from build123d import *

# Parameters (mm, degrees)
SKETCH_1_R      = 1.65
EXTRUDE_2_DEPTH = 2


with BuildPart() as part:
    # 草图1 → 凸台-拉伸2 (new body)
    with BuildSketch(Plane.XY):
        with BuildLine():
            ThreePointArc((64.930621202, 11.618442311), (61.467079618, -29.381557689), (64.930621202, -70.381557689))
            ThreePointArc((64.930621202, -70.381557689), (53.430621202, -81.881557689), (41.930621202, -70.381557689))
            ThreePointArc((41.930621202, -70.381557689), (45.394162787, -29.381557689), (41.930621202, 11.618442311))
            ThreePointArc((41.930621202, 11.618442311), (53.430621202, 23.118442311), (64.930621202, 11.618442311))
        make_face()
        with Locations((46.080621202, -70.381557689)):
            Circle(SKETCH_1_R, mode=Mode.SUBTRACT)
        with Locations((53.430621202, 4.268442311)):
            Circle(SKETCH_1_R, mode=Mode.SUBTRACT)
        with Locations((53.430621202, 11.618442311)):
            Circle(SKETCH_1_R, mode=Mode.SUBTRACT)
        with Locations((46.080621202, 11.618442311)):
            Circle(SKETCH_1_R, mode=Mode.SUBTRACT)
        with Locations((53.430621202, 18.968442311)):
            Circle(SKETCH_1_R, mode=Mode.SUBTRACT)
        with Locations((60.780621202, 11.618442311)):
            Circle(SKETCH_1_R, mode=Mode.SUBTRACT)
        with Locations((53.430621202, -70.381557689)):
            Circle(SKETCH_1_R, mode=Mode.SUBTRACT)
        with Locations((53.430621202, -63.031557689)):
            Circle(SKETCH_1_R, mode=Mode.SUBTRACT)
        with Locations((60.780621202, -70.381557689)):
            Circle(SKETCH_1_R, mode=Mode.SUBTRACT)
        with Locations((53.430621202, -77.731557689)):
            Circle(SKETCH_1_R, mode=Mode.SUBTRACT)
    extrude(amount=EXTRUDE_2_DEPTH)


solid = part.part
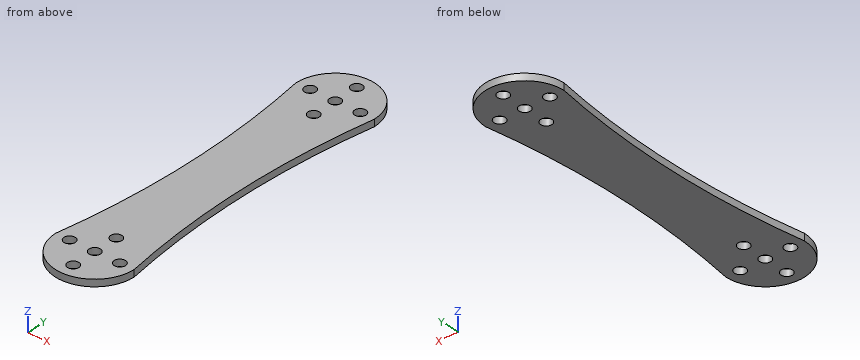
Geometry check sheet. Reference: the model listing, model coordinates, mm. Round coordinates to 2 decimals unless told otherwise and drop trailing zeros. Loops run counter-clockwise (first coordinate to the right, second up) from the corner with the lowest first, then second, coordinate; pieces in that order, holes last.
Item 1: Cross-section at C-C on y = -53. Record the boundary of the cut face in (x, z).
Item 2: Cross-section at A-A on x = 63.5. Record the boundary of the cut face in (y, z).
Item 3: Cross-section at B-B on z = 1.7. Count the separate pieces of the cut face and the enclosed holes in it, then the cut area to 3 significant figures.
Item 4: Gauge pin test, flat end, axial feed: pin 1 (1 mm diameter, centred on y = -49, z = 0.5, fed in from -X). Record the tip position at first contact, or that the pin passes through.
Item 5: Thickness scan on line 1 (Y direction, x = 59.5, z = 0.85); line 2 (Y direction, x = 60.5, z = 1.2); line 3 (X direction, y = -29.5, z = 0.7). Record the ranges inside material, lowest first.
Answer sheet:
1. outline: (44.25, 0) - (62.61, 0) - (62.61, 2) - (44.25, 2) - close
2. outline: (-75.94, 0) - (-60.84, 0) - (-60.84, 2) - (-75.94, 2) - close; (2.08, 0) - (17.17, 0) - (17.17, 2) - (2.08, 2) - close
3. separate pieces: 1
3. enclosed holes: 10
3. area: 1,840 mm2
4. pin 1: stops at x = 44.56
5. line 1: y = -80.15 to -71.42, -69.34 to 10.58, 12.66 to 21.39
5. line 2: y = -79.45 to -72.01, -68.76 to 9.99, 13.24 to 20.69
5. line 3: x = 45.39 to 61.47
